Work out the finished part from the listing and answer in its coordinate system (mm). A direction names the side the tool comes from. Round coordinates to 2 decimals unless told otherwise and drop trailing zeros. Write each loop counter-clockwise with the first axis right and the second up, starting at its lowest first coordinate (ties: lowest second). Pieces come first, ordered by that corner, then holes. Notation, with made-up numbers: (76.25, 3) - (103.25, 3) arc R35 cw to (103.25, 39) - close; hole circle Ø3 at (39.25, 29.5). An arc over 180 degrees is marked (long way). Write item = value, one per line. Start each with the question number.
from build123d import *

# Parameters (mm, degrees)
Y_KSEKLIK_EKSTR_ZYON1_DEPTH = 50
IZIM2_R                     = 7.5
Y_KSEKLIK_EKSTR_ZYON2_DEPTH = 10
RADYUS1_R                   = 10
PAH1_SIZE                   = 2


with BuildPart() as part:
    # Çizim1 → Yükseklik-Ekstrüzyon1 (new, symmetric)
    with BuildSketch(Plane.XY):
        with BuildLine():
            Line((-45.372360711, 120), (0, 0))
            Line((0, 0), (57.1, 0))
            Line((57.1, 0), (78.545069205, 10))
            Line((78.545069205, 10), (73.604661371, 23.960547839))
            ThreePointArc((73.604661371, 23.960547839), (63.364429783, 35.33825552), (48.078238331, 36.14257258))
            Line((48.078238331, 36.14257258), (16.591684434, 25))
            Line((16.591684434, 25), (-13.556112922, 110.191300263))
            ThreePointArc((-13.556112922, 110.191300263), (-23.989587023, 121.659965839), (-39.483672218, 122.22653082))
            Line((-39.483672218, 122.22653082), (-45.372360711, 120))
        make_face()
    extrude(amount=Y_KSEKLIK_EKSTR_ZYON1_DEPTH, both=True)

    # Çizim2 → Yükseklik-Ekstrüzyon2 (add)
    with BuildSketch(Plane.XZ):
        with Locations(Location((30, 0, 0), (0, 0, 90))):
            Circle(IZIM2_R)
    extrude(amount=Y_KSEKLIK_EKSTR_ZYON2_DEPTH)

    # Radyus1
    radyus1_edges = [part.edges().sort_by_distance(p)[0] for p in [
        (76.074865288, 16.980273919, -50),
        (-42.428016465, 121.11326541, -50),
        (76.074865288, 16.980273919, 50),
        (63.364429783, 35.33825552, 50),
        (32.334961383, 30.57128629, 50),
        (1.517785756, 67.595650131, 50),
        (-23.989587023, 121.659965839, 50),
        (-42.428016465, 121.11326541, 50),
        (-23.989587023, 121.659965839, -50),
        (1.517785756, 67.595650131, -50),
        (32.334961383, 30.57128629, -50),
        (63.364429783, 35.33825552, -50),
    ]]
    fillet(radyus1_edges, radius=RADYUS1_R)

    # Pah1
    pah1_edges = [part.edges().sort_by_distance(p)[0] for p in [
        (-20.917846504, 55.323142573, -50),
        (-20.917846504, 55.323142573, 50),
        (-45.372360711, 120, 0),
        (-44.336494724, 117.260360349, 47.071067812),
        (-44.336494724, 117.260360349, -47.071067812),
    ]]
    chamfer(pah1_edges, length=PAH1_SIZE)


solid = part.part
1. Find section C-C on y = 4. Give the vertices of the cut face in (x, z), plus the area to 3 significant figures.
2. Each of these flat-tipped pins is pushed along its axis until it touches: pin 1 (10 mm diameter, centred on y = 47.5, z = -22, fed in from -X); pin 2 (1 mm diameter, centred on x = 25, z = -11.5, fed in from +Y); pin 3 (1.5 mm diameter, centred on x = -26, z = 24, fed in from +Y); pin 4 (17 mm diameter, centred on x = 38.5, z = 1.5, fed in from -Y). Where does it stop, or does it pass through?
3. Find section B-B on z = 26.5. Give the vertices of the cut face in (x, y).
4. Find section A-A on z = 0. Give the vertices of the cut face in (x, y), plus the area to 3 significant figures.
5. For a pull along X with two mould halves and no side action, classify faces 1 (the face through (32.884, 27.576, -47.148)), 2 (the face through (-19.541, 54.549, 49.014)), 3 (the face through (-23.788, 121.565, 0.56)) as released by +X, released by -X, zero draft, split by the parting line, or undercut.
6. Consider line 1 (Y direction, x = 20.5, z = -28); line 2 (X direction, y = 11.5, z = 14); line 3 (Y direction, x = 71.5, z = 10). Determine where each line is inside the solid, lowest interval first.
7. Which of the six approach directions +Z, -Z, +X, -X, +Y, -Y give full straight-line access (tool end or side, diameter ignored) to faces 4 (the face through (0.117, 62.541, -47.148)), 5 (the face through (37.32, -4.93, -1.63)), 6 (the face through (0.117, 62.541, 47.148)), 7 (the face through (32.56, 30.65, 0.56)), 8 (the face through (-2, 40, -50))?
Answer key:
q1.outline = (-1.51, -48) - (0.63, -50) - (65.68, -50) - (65.68, 50) - (0.63, 50) - (-1.51, 48) - close
q1.area = 6,710 mm²
q2.pin_1 = -19.85
q2.pin_2 = 28.15
q2.pin_3 = 122.7
q2.pin_4 = -10
q3.outline = (-44.67, 118.13) - (0, 0) - (57.1, 0) - (78.55, 10) - (73.6, 23.96) arc R20 ccw to (48.08, 36.14) - (16.59, 25) - (-13.56, 110.19) arc R20 ccw to (-39.48, 122.23) - (-43.5, 120.71) - close
q4.outline = (-44.67, 118.13) - (0, 0) - (22.5, 0) - (22.5, -10) - (37.5, -10) - (37.5, 0) - (57.1, 0) - (78.55, 10) - (73.6, 23.96) arc R20 ccw to (48.08, 36.14) - (16.59, 25) - (-13.56, 110.19) arc R20 ccw to (-39.48, 122.23) - (-43.5, 120.71) - close
q4.area = 5,130 mm²
q5.face_1 = undercut
q5.face_2 = released by -X
q5.face_3 = split by the parting line
q6.line_1 = 0 to 26.38
q6.line_2 = -4.35 to 78.01
q6.line_3 = 6.71 to 28.22
q7.face_4 = -Z, +Y
q7.face_5 = -Y
q7.face_6 = +Z, +Y
q7.face_7 = +Z, -Z, +Y
q7.face_8 = -Z, +X, -X, +Y, -Y
